Input: part model. Units: mm. Frame: model coordinates. A direction names the side the tool comes from. Coordinates: 2 decimals unless noted, no trailing zeros. Write each loop counter-clockwise with the first axis right and the second up, starting at its lowest first coordinate (ties: lowest second). Pieces come first, ordered by that corner, then holes.
1) Section query A-A (z = -22). Output: boundary loops of the cut face in (x, y).
2) Section query C-C (z = -34.5). Output: boundary loops of the cut face in (x, y), then the cut area to 3 significant figures.
3) Draft query along Z for faces 4 (the flat face through (-3, -6.35, -2)), 5 (the flat face through (-43, -3, -41.81)), 6 (the flat face through (-28.115, -4.74, -0.176)). Return one class per face: pulls with the +Z half, pulls with the -Z half, needs draft (parallel to the pull), parting line crosses it, or undercut.
4) Pin query (flat end, axial travel): pin 1 Ø1 at (y, z) = (-2.5, 25) entering from +X; pin 2 Ø0.9 at (y, z) = (-3, -41.5) entering from -X; pin 3 Ø2.5 at (x, y) = (-53.5, -5) entering from +Z; pin 4 Ø4 at (x, z) = (14, 19) entering from +Y. Return the tip coordinate at first contact, or that it passes through.
5) Section query B-B (x = 2.5). Output: boundary loops of the cut face in (y, z).
6) Line query: L1, parallel to X at y = -0.25, z = 14.5; L2, parallel to Z at x = 18, y = -2; L3, parallel to X at y = -3.75, z = -29. Output: solid intervals per line, ascending.
7) Set-up query: faces 1 (the flat face through (-29, -3.175, -3)), 2 (the flat face through (-46.589, -4.74, -10.327)), 3 (the flat face through (-23.873, -3.131, -34.192)). Return all of +Z, -Z, +X, -X, +Y, -Y with unobstructed straight access to the full face (end or side cutting, diameter ignored); none if empty.
from build123d import *

# Parameters (mm, degrees)
F1_DEPTH = 6.35
F3_DEPTH = 6.351
F5_DEPTH = 3.175
F6_W     = 12.7
F6_H     = 6.35
F7_DEPTH = 0.79375


with BuildPart() as f1:
    # F0 (on Front) → F1 (new body)
    with BuildSketch(Plane.XZ):
        with BuildLine():
            Line((-24.499685, 6.084885), (-31.832033, -6.615115))
            Line((-31.832033, -6.615115), (-32.680925, -10.581826))
            Line((-32.680925, -10.581826), (-51.059928, -7.35622))
            Line((-51.059928, -7.35622), (-56.454085, -7.35622))
            Line((-56.454085, -7.35622), (-56.454085, -7.889269))
            Line((-56.454085, -7.889269), (-36.444739, -12.834284))
            Line((-36.444739, -12.834284), (-42.707812, -18.690551))
            ThreePointArc((-42.707812, -18.690551), (-45.886659, -22.415252), (-48.779547, -26.366159))
            Line((-48.779547, -26.366159), (-50.759438, -31.151975))
            ThreePointArc((-50.759438, -31.151975), (-49.034652, -31.438473), (-47.444712, -30.711107))
            Line((-47.444712, -30.711107), (-33.90066, -18.69024))
            Line((-33.90066, -18.69024), (-48.100285, -39.247155))
            Line((-48.100285, -39.247155), (-52.266728, -49.726259))
            Line((-52.266728, -49.726259), (-49.289104, -51.483847))
            ThreePointArc((-49.289104, -51.483847), (-47.937249, -51.364421), (-46.760015, -50.68922))
            Line((-46.760015, -50.68922), (-33.575531, -38.721569))
            Line((-33.575531, -38.721569), (-30.814609, -40.181708))
            ThreePointArc((-30.814609, -40.181708), (-24.988749, -38.958576), (-20.071417, -35.603501))
            Line((-20.071417, -35.603501), (-27.781654, -32.740546))
            Line((-27.781654, -32.740546), (-13.891757, -19.627586))
            ThreePointArc((-13.891757, -19.627586), (-10.881214, -17.587078), (-7.379708, -16.603975))
            Line((-7.379708, -16.603975), (8.157321, -16.091641))
            ThreePointArc((8.157321, -16.091641), (10.488998, -15.52545), (12.401008, -14.075792))
            Line((12.401008, -14.075792), (18.136641, -7.494206))
            Line((18.136641, -7.494206), (44.15147, -1.607402))
            ThreePointArc((44.15147, -1.607402), (48.239493, -0.096798), (51.586218, 2.694848))
            ThreePointArc((51.586218, 2.694848), (51.877375, 3.698296), (51.586218, 4.701744))
            ThreePointArc((51.586218, 4.701744), (47.456215, 7.294304), (42.746603, 8.558366))
            Line((42.746603, 8.558366), (26.455848, 10.407886))
            Line((26.455848, 10.407886), (23.768522, 11.395085))
            Line((23.768522, 11.395085), (23.636915, 15.313192))
            Line((23.636915, 15.313192), (11.526386, 14.906407))
            Line((11.526386, 14.906407), (13.124879, 22.049895))
            Line((13.124879, 22.049895), (20.507815, 24.478994))
            Line((20.507815, 24.478994), (20.507815, 25.678071))
            Line((20.507815, 25.678071), (13.484901, 26.78713))
            Line((13.484901, 26.78713), (15.122742, 37.158459))
            ThreePointArc((15.122742, 37.158459), (9.02504, 35.504795), (4.668364, 30.929212))
            ThreePointArc((4.668364, 30.929212), (0.413088, 27.492182), (-3.282097, 23.459049))
            Line((-3.282097, 23.459049), (-12.800315, 11.367148))
            Line((-12.800315, 11.367148), (-10.821415, 19.223839))
            Line((-10.821415, 19.223839), (-11.518751, 20.283149))
            Line((-11.518751, 20.283149), (-16.865773, 16.763244))
            Line((-16.865773, 16.763244), (-25.769467, 30.28868))
            Line((-25.769467, 30.28868), (-29.317735, 28.515689))
            Line((-29.317735, 28.515689), (-24.499685, 6.084885))
        make_face()
    extrude(amount=F1_DEPTH)

    # F2 (on face) → F3 (cut, through all)
    with BuildSketch(Plane.XZ.offset(6.35)):
        Polygon((-36.103749, -51.509792), (-36.103749, -41.01645), (-48.803749, -41.01645), (-61.503749, -41.01645), (-61.503749, -51.509792), align=None)
    extrude(amount=-F3_DEPTH, mode=Mode.SUBTRACT)

    # F4 (on face) → F5 (cut)
    with BuildSketch(Plane(origin=(0, 0, 0), x_dir=(-1, 0, 0), z_dir=(0, 1, 0))):
        Polygon((56.454085, 11.32442), (14.556029, 10.607801), (29.449862, -15.189074), (56.454085, -15.905692), align=None)
    extrude(amount=-F5_DEPTH, mode=Mode.SUBTRACT)

    # F6 (on face) → F7 (join)
    with BuildSketch(Plane(origin=(0, 0, -41.01645), x_dir=(1, 0, 0), z_dir=(0, 0, -1))):
        with Locations((-42.453749, 3.175)):
            Rectangle(F6_W, F6_H)
    extrude(amount=F7_DEPTH)


solid = f1.part
Answer:
1. outline: (-45.56, -6.35) - (-37.63, -6.35) - (-37.63, 0) - (-45.56, 0) - close; (-36.19, -6.35) - (-16.4, -6.35) - (-16.4, 0) - (-36.19, 0) - close
2. outline: (-44.82, -6.35) - (-23.04, -6.35) - (-23.04, 0) - (-44.82, 0) - close
2. area: 138 mm2
3. face 4: needs draft
3. face 5: pulls with the -Z half
3. face 6: undercut
4. pin 1: stops at x = 20.51
4. pin 2: stops at x = -48.8
4. pin 3: stops at z = -7.36
4. pin 4: stops at y = 0
5. outline: (-6.35, -16.28) - (0, -16.28) - (0, 29.31) - (-6.35, 29.31) - close
6. L1: x = -26.31 to -12.01, -10.33 to 23.66
6. L2: z = -7.65 to 15.12, 23.65 to 26.07
6. L3: x = -49.87 to -45.52, -41.02 to -23.82
7. face 1: -X, +Y
7. face 2: -X, +Y, -Y
7. face 3: +X, +Y, -Y
